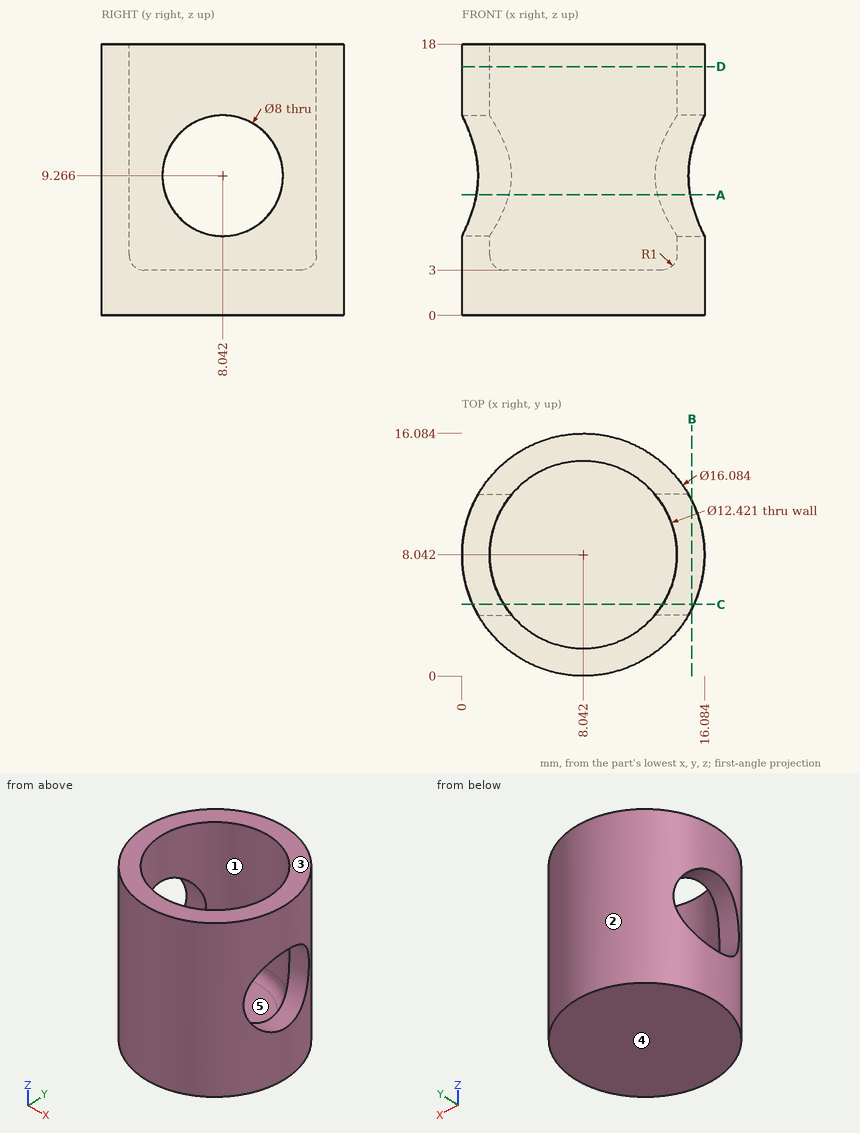
Geometry check sheet. Reference: drawing and pictorial views, mm from the part's lowest x, y, z. A direction names the side the tool comes from. Round coordinates to 2 decimals unless told otherwise and drop trailing zeros. Write each loop counter-clockwise with the first axis right and the second up, starting at its lowest first coordinate (ties: lowest second). Pieces come first, ordered by that corner, then holes.
Item 1: Section check B-B (x = 15.25). Record the boundary of the cut face in (y, z) (1 decimal).
Determined:
outline: (4.5, 0) - (11.6, 0) - (11.6, 7.5) arc R4 cw to (4.5, 7.5) - close; (4.5, 11.1) arc R4 cw to (11.6, 11.1) - (11.6, 18) - (4.5, 18) - close
Item 2: Section check A-A (z = 8). Record the boundary of the cut face in (x, y) (1 decimal).
Determined:
outline: (1, 4.2) arc R8 ccw to (15.1, 4.2) - (13, 4.2) arc R6.2 cw to (3.1, 4.2) - close; (1, 11.8) - (3.1, 11.8) arc R6.2 cw to (13, 11.8) - (15.1, 11.8) arc R8 ccw to start
Item 3: Section check D-D (z = 16.5). Record the boundary of the cut face in (x, y) (1 decimal).
Determined:
outline: circle Ø16.1 at (8, 8); hole circle Ø12.4 at (8, 8)
Item 4: Mould release check, pull along X, two halves, no side actions. Record for the marked faces 1, 2 and 3: +X half, -X half, draft (parallel to the pull), parting line (faces both ways), or undercut.
Determined:
face 1: undercut
face 2: parting line
face 3: draft
Item 5: Material ranges on line 1 along Z through (x, y) = (1, 11.5) (1 decimal); line 2 along X through (y, z) = (11, 16) (1 decimal); line 3 along X through (y, z) = (6, 13.75) (1 decimal), recorded low to high.
Determined:
line 1: z = 0 to 7.3, 11.3 to 18
line 2: x = 0.6 to 2.6, 13.5 to 15.5
line 3: x = 0.3 to 2.2, 13.9 to 15.8
Item 6: Access from +Z, -Z, +X, -X, +Y, -Y to the whole of each face (thin tool, end or side, straight path). Record for the marked faces 4 and 5.
Determined:
face 4: -Z, +X, -X, +Y, -Y
face 5: +Z
Item 7: Section check C-C (y = 4.75). Give the number of separate pieces and of enclosed holes in the cut face.
Determined:
separate pieces: 3
enclosed holes: 0
Item 8: Go/stop test with flat-tipped pins: pin 1 Ø5 at (x, z) = (12, 5) entering from -Y; pin 2 Ø3 at (x, y) = (9.5, 10) entering from +Z; pin 3 Ø1.5 at (x, z) = (2.5, 6) entering from +Y. Record where each tip stops, or that it passes through.
Determined:
pin 1: stops at y = 0.13
pin 2: stops at z = 3
pin 3: stops at y = 14.5
